Can you work these out from the model? Positions are in its coordinate system, mm. Face numbers are marked on the shaded views. A direction names the side the tool comes from. Round coordinates to 2 decimals unless told otherwise and drop trailing zeros. Write each loop counter-clockwise with the first axis right and the second up, starting at its lowest first coordinate (ties: lowest second). Pieces come first, ordered by that corner, then holes. Notation, with made-up numbers: M -30,9 L 12,9 A18 ccw 12,20 Z; hole C -1.75,72.5 d8. An arc over 180 degrees is marked long. Answer in a Markdown table with one row per item. Add a question column.
(1) Suppose I cut it at B-B, the plane x = -53. Write out the boundary of the cut face in (y, z), then the cut area to 3 significant figures.
(2) I'm going to push a flat-ended pin straight in: pin 1 (1.1 mm diameter, centred on y = 2.5, z = 32.5, fed in from +X). Where does the tip first touch, or does it pass through?
(3) Suppose I cut it at A-A, the plane z = 3.81. Write out the boundary of the cut face in (x, y), then the cut area to 3 significant figures.
(4) If I drill on probe 1 along X at (y, z) = (0.65, 3.81); probe 2 along X at (y, z) = (2.05, 3.81); probe 3 along X at (y, z) = (2.3, 62), over which ranges is the centre line in solid material (lowest first)?
(5) For the marked faces 1 and 2, which set-ups out of +Z, -Z, +X, -X, +Y, -Y let a thin tool reach every point of the face, with its end or its side?
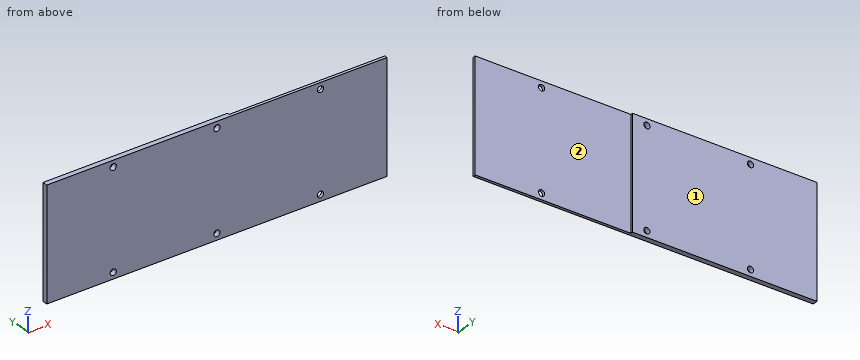
Autodesk Inventor part; units mm, degrees
ref_plane "YZ Plane" through (0, 0, 0) normal (1, 0, 0) x (0, 1, 0)
ref_plane "XZ Plane" through (0, 0, 0) normal (0, 1, 0) x (-1, 0, 0)
ref_plane "XY Plane" through (0, 0, 0) normal (0, 0, 1) x (1, 0, 0)
sketch "Sketch1" plane through (0, 0, 0) normal (0, 1, 0) x (-1, 0, 0)
  line L0 (0, 0) -> (200.152, 0)
  line L1 (200.152, 0) -> (200.152, 66.1924)
  line L2 (200.152, 66.1924) -> (0, 66.1924)
  line L3 (0, 66.1924) -> (0, 0)
  dimension "d0" = 66.1924
  dimension "d1" = 200.152
extrude "Extrusion1" add sketch "Sketch1" along normal blind 3.048
sketch "Sketch2" plane through (0, 3.048, 0) normal (0, 1, 0) x (1, 0, 0)
  line L0 (-200.152, -66.1924) -> (0, -66.1924)
  line L1 (-100.076, -66.1924) -> (-100.076, 0) construction
  line L2 (0, 0) -> (-200.152, 0)
  point P0 (-100.076, -62.3824)
  point P1 (-100.076, -3.81)
  point P2 (-39.116, -62.3824)
  point P3 (-39.116, -3.81)
  point P4 (-161.036, -3.81)
  point P5 (-161.036, -62.3824)
  dimension "d4" = 3.81
  dimension "d5" = 3.81
  dimension "d6" = 60.96
  dimension "d7" = 60.96
hole "Hole1" at (-100.076, 3.048, 62.3824) at (-100.076, 3.048, 3.81) at (-39.116, 3.048, 62.3824) at (-39.116, 3.048, 3.81) at (-161.036, 3.048, 3.81) at (-161.036, 3.048, 62.3824) direction (0, -1, 0) diameter 3.6576 end through all
sketch "Sketch3" plane through (0, 3.048, 0) normal (0, 1, 0) x (1, 0, 0)
  line L0 (0, -66.1924) -> (0, 0)
  line L1 (0, -66.1924) -> (-91.6178, -66.1924)
  line L2 (-91.6178, -66.1924) -> (-91.6178, 0)
  line L3 (-91.6178, 0) -> (0, 0)
  line L4 (0, 0) -> (0, -66.1924)
  line L5 (0, 0) -> (-200.152, 0)
  point P0 (-100.076, 0)
  dimension "d15" = 8.4582
extrude "Extrusion2" cut sketch "Sketch3" against normal blind 1.3208
properties part number "TopLayerPlate"
Calculated:
| question | item | result |
|---|---|---|
| 1 | outline | M 0,0 L 1.73,0 L 1.73,66.19 L 0,66.19 Z |
| 1 | area | 114 mm² |
| 2 | pin 1 | x = -91.62 |
| 3 | outline | M -200.15,0 L -162.86,0 L -162.86,3.05 L -200.15,3.05 Z; M -159.21,0 L -101.9,0 L -101.9,3.05 L -159.21,3.05 Z; M -98.25,0 L -40.94,0 L -40.94,1.73 L -91.62,1.73 L -91.62,3.05 L -98.25,3.05 Z; M -37.29,0 L 0,0 L 0,1.73 L -37.29,1.73 Z |
| 3 | area | 460 mm² |
| 4 | probe 1 | -200.15 to -162.86, -159.21 to -101.9, -98.25 to -40.94, -37.29 to 0 |
| 4 | probe 2 | -200.15 to -162.86, -159.21 to -101.9, -98.25 to -91.62 |
| 4 | probe 3 | -200.15 to -162.82, -159.25 to -101.86, -98.29 to -91.62 |
| 5 | face 1 | +Z, -Z, +X, -X, +Y |
| 5 | face 2 | +Z, -Z, +X, +Y |
